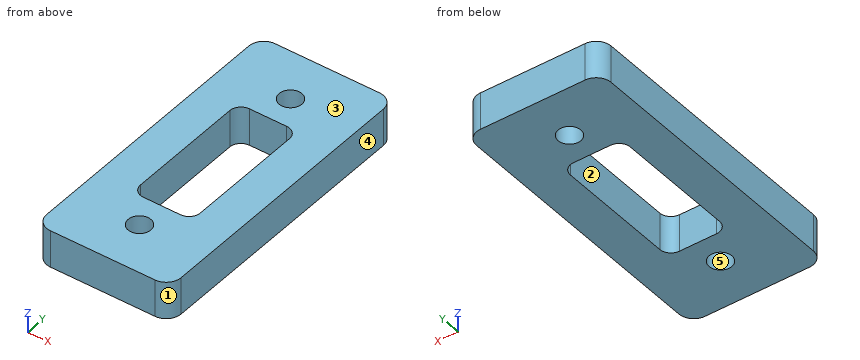
from build123d import *

# Parameters (mm, degrees)
SKETCH_1_W          = 18
SKETCH_1_H          = 40
SKETCH_1_R          = 1.525
EXTRUDE_1_DEPTH     = 5
FILLET_1_R          = 2
SKETCH_2_W          = 8
SKETCH_2_H          = 18.9
CUT_EXTRUDE_1_DEPTH = 5
FILLET_2_R          = 1.5


with BuildPart() as part:
    # 草图1 → 凸台-拉伸1 (new body)
    with BuildSketch(Plane.XY):
        Rectangle(SKETCH_1_W, SKETCH_1_H)
        with Locations((0, 13.45)):
            Circle(SKETCH_1_R, mode=Mode.SUBTRACT)
        with Locations((0, -13.45)):
            Circle(SKETCH_1_R, mode=Mode.SUBTRACT)
    extrude(amount=EXTRUDE_1_DEPTH)

    # 圆角1
    fillet_1_edges = [part.edges().sort_by_distance(p)[0] for p in [
        (9, -20, 2.5),
        (-9, -20, 2.5),
        (-9, 20, 2.5),
        (9, 20, 2.5),
    ]]
    fillet(fillet_1_edges, radius=FILLET_1_R)

    # 草图2 → 切除-拉伸1 (cut)
    with BuildSketch(Plane.XY.offset(5)):
        Rectangle(SKETCH_2_W, SKETCH_2_H)
    extrude(amount=-CUT_EXTRUDE_1_DEPTH, mode=Mode.SUBTRACT)

    # 圆角2
    fillet_2_edges = [part.edges().sort_by_distance(p)[0] for p in [
        (4, 9.45, 2.5),
        (4, -9.45, 2.5),
        (-4, -9.45, 2.5),
        (-4, 9.45, 2.5),
    ]]
    fillet(fillet_2_edges, radius=FILLET_2_R)


solid = part.part
Part model, mm, in its own coordinate system. Face numbers are marked on the shaded views. A direction names the side the tool comes from. Coordinates: 2 decimals unless noted, no trailing zeros. Order: outer loops, then holes, each group sorted by start corner. A loop starts at its lowest first (then second) coordinate and runs counter-clockwise, first axis right, second up.
(1) Tool access for the marked faces 1 and 2: list every direction of +Z, -Z, +X, -X, +Y, -Y with a clear straight run to the whole face (end or side of a thin tool).
Check sheet entries:
face 1: +Z, -Z, +X, -Y
face 2: +Z, -Z
(2) Slice it at A-A, the plane y = -13.45. Write the cut outline in (x, z) (3 decimals).
Check sheet entries:
outline: (-9, 0) - (-1.525, 0) - (-1.525, 5) - (-9, 5) - close; (1.525, 0) - (9, 0) - (9, 5) - (1.525, 5) - close
(3) Pull direction X, two halves, no side cores. Call the marked faces 3, 4 and 5: pulls with the +X half, pulls with the -X half, needs draft (parallel to the pull), parting line crosses it, or undercut.
Check sheet entries:
face 3: needs draft
face 4: pulls with the +X half
face 5: undercut
(4) Probe L1, parallel to X at y = 3.5, z = 2.2; L2, parallel to Y at x = 1.25, z = 2.9; L3, parallel to Y at x = -2.75, z = 3.25. List the from-to ranges inside material, lowest first.
Check sheet entries:
L1: x = -9 to -4, 4 to 9
L2: y = -20 to -14.32, -12.58 to -9.45, 9.45 to 12.58, 14.32 to 20
L3: y = -20 to -9.43, 9.43 to 20
(5) Slice it at C-C, the plane z = 2.5. Write the cut outline in (x, y) (3 decimals), and give its area (3 significant figures).
Check sheet entries:
outline: (-9, -18) arc R2 ccw to (-7, -20) - (7, -20) arc R2 ccw to (9, -18) - (9, 18) arc R2 ccw to (7, 20) - (-7, 20) arc R2 ccw to (-9, 18) - close; hole (-4, -7.95) arc R1.5 ccw to (-2.5, -9.45) - (2.5, -9.45) arc R1.5 ccw to (4, -7.95) - (4, 7.95) arc R1.5 ccw to (2.5, 9.45) - (-2.5, 9.45) arc R1.5 ccw to (-4, 7.95) - close; hole circle Ø3.05 at (0, -13.45); hole circle Ø3.05 at (0, 13.45)
area: 553 mm2
(6) Slice it at B-B, the plane x = 0. Write the cut outline in (y, z) (3 decimals), and give its area (3 significant figures).
Check sheet entries:
outline: (-20, 0) - (-14.975, 0) - (-14.975, 5) - (-20, 5) - close; (-11.925, 0) - (-9.45, 0) - (-9.45, 5) - (-11.925, 5) - close; (9.45, 0) - (11.925, 0) - (11.925, 5) - (9.45, 5) - close; (14.975, 0) - (20, 0) - (20, 5) - (14.975, 5) - close
area: 75.0 mm2
(7) Pin check, flat tips, straight feed: pin 1 Ø3 at (x, y) = (3.5, -7) entering from +Z; pin 2 Ø2.5 at (x, y) = (0, 13.45) entering from +Z. Stop position of each tip, or through.
Check sheet entries:
pin 1: stops at z = 5
pin 2: passes through
(8) Slice it at D-D, the plane y = 14.5. Write the cut outline in (x, z).
Check sheet entries:
outline: (-9, 0) - (-1.11, 0) - (-1.11, 5) - (-9, 5) - close; (1.11, 0) - (9, 0) - (9, 5) - (1.11, 5) - close
